Geometry check sheet. Reference: the model listing, model coordinates, mm. A direction names the side the tool comes from. Round coordinates to 2 decimals unless told otherwise and drop trailing zeros. Loops run counter-clockwise (first coordinate to the right, second up) from the corner with the lowest first, then second, coordinate; pieces in that order, holes last. Notation, with made-up numbers: (-14.75, 51) -> (22.25, 51) arc R19 cw to (22.25, 63) -> close; hole circle Ø8 at (-31.5, 21). An arc over 180 degrees is marked (long way). Use one line per item in the form item = value.
from build123d import *

# Parameters (mm, degrees)
F2_DEPTH      = 200
F2_DEPTH_BACK = 200
F4_DEPTH      = 4000


with BuildPart() as f2:
    # F1 (on face) → F2 (new body, two sides)
    with BuildSketch(Plane.XZ) as f2_sk:
        with BuildLine():
            Line((-400, -200), (400, -200))
            ThreePointArc((400, -200), (600, 0), (400, 200))
            Line((400, 200), (-400, 200))
            ThreePointArc((-400, 200), (-600, 0), (-400, -200))
        make_face()
    extrude(amount=-F2_DEPTH)
    extrude(f2_sk.sketch, amount=F2_DEPTH_BACK)

    # F3 (on face) → F4 (cut)
    with BuildSketch(Plane.XZ.offset(200)):
        with BuildLine():
            Line((-400, -150), (400, -150))
            ThreePointArc((400, -150), (550, 0), (400, 150))
            Line((400, 150), (-400, 150))
            ThreePointArc((-400, 150), (-550, 0), (-400, -150))
        make_face()
    extrude(amount=-F4_DEPTH, mode=Mode.SUBTRACT)


solid = f2.part
1. Section check C-C (y = 167). Record the boundary of the cut face in (x, z).
Return value:
outline = (-400, -200) -> (400, -200) arc R200 ccw to (400, 200) -> (-400, 200) arc R200 ccw to start; hole (-400, -150) -> (400, -150) arc R150 ccw to (400, 150) -> (-400, 150) arc R150 ccw to start
2. Tool access check on faces 1 (the flat face through (42, 200, 164)), 2 (the flat face through (6, -3, 150)). Record the directions out of +Z, -Z, +X, -X, +Y, -Y that give a thin tool (end or side, any length) a straight path to the whole face; none if there is none.
Return value:
face_1 = +Z, -Z, +X, -X, +Y
face_2 = +Y, -Y
3. Material ranges on line 1 along Z through (x, y) = (-368, 43); line 2 along X through (y, z) = (-36.5, -2); line 3 along X through (y, z) = (107.5, -14.5), recorded low to high.
Return value:
line_1 = -200 to -150, 150 to 200
line_2 = -599.99 to -549.99, 549.99 to 599.99
line_3 = -599.47 to -549.3, 549.3 to 599.47
4. Mould release check, pull along X, two halves, no side actions. Record for faces 3 (the flat face through (6, 3, 200)), 4 (the cylindrical face through (-599.95, 2.8, 4.4)), 5 (the flat face through (-6, -3, -150)): released by +X, released by -X, zero draft, split by the parting line, or undercut.
Return value:
face_3 = zero draft
face_4 = released by -X
face_5 = undercut
5. Gauge pin test, flat ends, axial feed: pin 1 (12 mm diameter, centred on y = -106, z = -44.5, fed in from -X); pin 2 (10 mm diameter, centred on y = 58.5, z = 126, fed in from +X); pin 3 (6 mm diameter, centred on y = 97.5, z = 26.5, fed in from +X). Record the tip position at first contact, or that the pin passes through.
Return value:
pin_1 = -596.26
pin_2 = 559.25
pin_3 = 598.61
6. Section check B-B (x = 232.5). Record the boundary of the cut face in (y, z).
Return value:
outline = (-200, -200) -> (200, -200) -> (200, -150) -> (-200, -150) -> close; (-200, 150) -> (200, 150) -> (200, 200) -> (-200, 200) -> close
7. Section check D-D (z = 169). Record the boundary of the cut face in (x, y), then the cut area to 3 significant figures.
Return value:
outline = (-506.95, -200) -> (506.95, -200) -> (506.95, 200) -> (-506.95, 200) -> close
area = 406,000 mm2
8. Section check A-A (z = 0). Record the boundary of the cut face in (x, y), then the cut area to 3 significant figures.
Return value:
outline = (-600, -200) -> (-550, -200) -> (-550, 200) -> (-600, 200) -> close; (550, -200) -> (600, -200) -> (600, 200) -> (550, 200) -> close
area = 40,000 mm2
